from build123d import *

# Parameters (mm, degrees)
SKETCH_1_R          = 3
EXTRUDE_1_DEPTH     = 13
SKETCH_2_R          = 2.5
EXTRUDE_2_DEPTH     = 5
SKETCH_3_W          = 1.5
SKETCH_3_H          = 7.126757192
CUT_EXTRUDE_1_DEPTH = 1


with BuildPart() as part:
    # Эскиз1 → Бобышка-Вытянуть1 (new body)
    with BuildSketch(Plane.XY):
        with Locations(Location((0, 0, 0), (0, 0, 180))):
            Circle(SKETCH_1_R)
    extrude(amount=EXTRUDE_1_DEPTH)

    # Эскиз2 → Бобышка-Вытянуть2 (add)
    with BuildSketch(Plane.XY.offset(13)):
        Circle(SKETCH_2_R)
    extrude(amount=EXTRUDE_2_DEPTH)

    # Эскиз3 → Вырез-Вытянуть1 (cut)
    with BuildSketch(Plane(origin=(0, 0, 0), x_dir=(-1, 0, 0), z_dir=(0, 0, -1))):
        with Locations((0, 0.049491369)):
            Rectangle(SKETCH_3_W, SKETCH_3_H)
    extrude(amount=-CUT_EXTRUDE_1_DEPTH, mode=Mode.SUBTRACT)


solid = part.part
Can you work these out from the model? Positions are in its coordinate system, mm. A direction names the side the tool comes from. Coordinates: 2 decimals unless noted, no trailing zeros. Order: outer loops, then holes, each group sorted by start corner. A loop starts at its lowest first (then second) coordinate and runs counter-clockwise, first axis right, second up. Notation, with made-up numbers: M -39.75,11 L -15.75,11 A26 ccw -15.75,30 Z; hole C -4,14 d3. An arc over 180 degrees is marked long. Write item = value, one per line.
(1) For faces 1 (the face through (-2.77, 1.15, 6.41)), 2 (the face through (-0.54, -2.44, 15.46)), 3 (the face through (0, 0, 1)), which set-ups out of +Z, -Z, +X, -X, +Y, -Y let a thin tool reach every point of the face, with its end or its side?
Results are:
face_1 = +Z, -Z
face_2 = +Z
face_3 = -Z, +Y, -Y
(2) Suppose I cut it at D-D on x = -2. Please give me the cut outline in (y, z), plus the area to 3 significant figures.
Results are:
outline = M -2.24,0 L 2.24,0 L 2.24,13 L 1.5,13 L 1.5,18 L -1.5,18 L -1.5,13 L -2.24,13 Z
area = 73.1 mm2
(3) Suppose I cut it at A-A on x = 0. Please give me the cut outline in (y, z), plus the area to 3 significant figures.
Results are:
outline = M -3,1 L 3,1 L 3,13 L 2.5,13 L 2.5,18 L -2.5,18 L -2.5,13 L -3,13 Z
area = 97.0 mm2
(4) For pin 1 Ø0.5 at (x, y) = (0, 1) entering from -Z; pin 2 Ø1.5 at (y, z) = (-0.5, 11) entering from +X; pin 3 Ø0.5 at (y, z) = (1, 0.5) entering from -X; pin 4 Ø1.5 at (x, z) = (1, 15.5) entering from +Y, each with a flat end and sliding along its axis, tell me the tip position at first contact or that it passes through.
Results are:
pin_1 = 1
pin_2 = 3
pin_3 = -2.9
pin_4 = 2.49
(5) Suppose I cut it at C-C on z = 13.5. Please give me the cut outline in (x, y).
Results are:
outline = C 0,0 d5
(6) I need wall thicknesses on line 1 along X through (y, z) = (0.15, 16.5); line 2 along Z through (x, y) = (0.35, 1.55); line 3 along X through (y, z) = (0.75, 10.25). Which ranges of each line are inside material? Lowest first, please. Write a range as [from, to].
Results are:
line_1 = [-2.5, 2.5]
line_2 = [1, 18]
line_3 = [-2.9, 2.9]
(7) Suppose I cut it at B-B on y = 0.2. Please give me the cut outline in (x, z).
Results are:
outline = M -2.99,0 L -0.75,0 L -0.75,1 L 0.75,1 L 0.75,0 L 2.99,0 L 2.99,13 L 2.49,13 L 2.49,18 L -2.49,18 L -2.49,13 L -2.99,13 Z
